from build123d import *

# Parameters (mm, degrees)
SKETCH1_W           = 30
SKETCH1_H           = 29
BOSS_EXTRUDE1_DEPTH = 10
SKETCH2_W           = 4
SKETCH2_H           = 10
CUT_EXTRUDE1_DEPTH  = 10
CHAMFER1_SIZE       = 4
SKETCH3_R           = 2
CUT_EXTRUDE2_DEPTH  = 15
CHAMFER2_SIZE       = 0.5
SKETCH4_R           = 10
CUT_EXTRUDE3_DEPTH  = 24.135470603
BOSS_EXTRUDE2_DEPTH = 19
CHAMFER3_SIZE       = 4
SKETCH6_W           = 28
SKETCH6_H           = 10
CUT_EXTRUDE4_DEPTH  = 15
FILLET1_R           = 5
SKETCH7_R           = 1.75
CUT_EXTRUDE5_DEPTH  = 69.85245211
FILLET2_R           = 2
SKETCH8_R           = 2
CUT_EXTRUDE6_DEPTH  = 61.478592634
SKETCH9_R           = 7.5
CUT_EXTRUDE7_DEPTH  = 5
BOSS_EXTRUDE3_DEPTH = 5


with BuildPart() as part:
    # Sketch1 → Boss-Extrude1 (new body)
    with BuildSketch(Plane.XY):
        Rectangle(SKETCH1_W, SKETCH1_H)
    extrude(amount=BOSS_EXTRUDE1_DEPTH)

    # Sketch2 → Cut-Extrude1 (cut)
    with BuildSketch(Plane.XZ.offset(14.5)):
        with Locations((-13, 5)):
            Rectangle(SKETCH2_W, SKETCH2_H)
        with Locations((13, 5)):
            Rectangle(SKETCH2_W, SKETCH2_H)
    extrude(amount=-CUT_EXTRUDE1_DEPTH, mode=Mode.SUBTRACT)

    # Chamfer1
    chamfer1_edges = [part.edges().sort_by_distance(p)[0] for p in [
        (11, -4.5, 5),
        (-11, -4.5, 5),
    ]]
    chamfer(chamfer1_edges, length=CHAMFER1_SIZE - 0.0001)  # a hair under: the kernel refuses the full size

    # Sketch3 → Cut-Extrude2 (cut)
    with BuildSketch(Plane.XZ.offset(14.5)):
        with Locations(Location((-7.5, 5, 0), (0, 0, 270))):
            Circle(SKETCH3_R)
        with Locations(Location((0, 5, 0), (0, 0, 270))):
            Circle(SKETCH3_R)
        with Locations(Location((7.5, 5, 0), (0, 0, 270))):
            Circle(SKETCH3_R)
    extrude(amount=-CUT_EXTRUDE2_DEPTH, mode=Mode.SUBTRACT)

    # Chamfer2
    chamfer2_edges = [part.edges().sort_by_distance(p)[0] for p in [
        (-7.5, -14.5, 7),
        (0, -14.5, 7),
        (7.5, -14.5, 7),
    ]]
    chamfer(chamfer2_edges, length=CHAMFER2_SIZE)

    # Sketch4 → Cut-Extrude3 (cut, through all)
    with BuildSketch(Plane(origin=(0, 0, 0), x_dir=(-1, 0, 0), z_dir=(0, 0, -1))):
        with Locations((0, -2.5)):
            Circle(SKETCH4_R)
    extrude(amount=-CUT_EXTRUDE3_DEPTH, mode=Mode.SUBTRACT)

    # Sketch5 → Boss-Extrude2 (add, symmetric)
    with BuildSketch(Plane(origin=(0, 0, 0), x_dir=(0, 0, -1), z_dir=(1, 0, 0))):
        Polygon((-10, 13.5), (-27.320508076, 23.5), (-27.320508076, 50.5), (-17.320508076, 50.5), (-17.320508076, 24.5), (0, 14.5), align=None)
    extrude(amount=BOSS_EXTRUDE2_DEPTH, both=True)

    # Chamfer3
    chamfer3_edges = [part.edges().sort_by_distance(p)[0] for p in [
        (-19, 14, 5),
        (19, 14, 5),
    ]]
    chamfer(chamfer3_edges, length=CHAMFER3_SIZE - 0.0001)  # a hair under: the kernel refuses the full size

    # Sketch6 → Cut-Extrude4 (cut)
    with BuildSketch(Plane(origin=(0, 50.5, 0), x_dir=(1, 0, 0), z_dir=(0, 1, 0))):
        with Locations((0, -22.320508076)):
            Rectangle(SKETCH6_W, SKETCH6_H)
    extrude(amount=-CUT_EXTRUDE4_DEPTH, mode=Mode.SUBTRACT)

    # Fillet1
    fillet1_edges = [part.edges().sort_by_distance(p)[0] for p in [
        (16.5, 50.5, 17.320508076),
        (16.5, 50.5, 27.320508076),
        (-16.5, 50.5, 17.320508076),
        (-16.5, 50.5, 27.320508076),
    ]]
    fillet(fillet1_edges, radius=FILLET1_R - 0.0001)  # a hair under: the kernel refuses the full size

    # Sketch7 → Cut-Extrude5 (cut, through all)
    with BuildSketch(Plane(origin=(19, 0, 0), x_dir=(0, 0, -1), z_dir=(1, 0, 0))):
        with Locations((-22.320508076, 45.5)):
            Circle(SKETCH7_R)
    extrude(amount=-CUT_EXTRUDE5_DEPTH, mode=Mode.SUBTRACT)

    # Fillet2
    fillet2_edges = [part.edges().sort_by_distance(p)[0] for p in [
        (19, 34.50005, 27.320508076),
        (19, 49.035563195, 25.856071271),
        (19, 49.035563195, 18.78494488),
        (-19, 34.50005, 27.320508076),
        (-19, 49.035563195, 25.856071271),
        (-19, 49.035563195, 18.78494488),
        (-19, 35.00005, 17.320508076),
        (19, 35.00005, 17.320508076),
    ]]
    fillet(fillet2_edges, radius=FILLET2_R)

    # Sketch8 → Cut-Extrude6 (cut, through all)
    with BuildSketch(Plane.XY.offset(27.320508076)):
        with Locations((0, 30.5)):
            Circle(SKETCH8_R)
    extrude(amount=-CUT_EXTRUDE6_DEPTH, mode=Mode.SUBTRACT)

    # Sketch9 → Cut-Extrude7 (cut)
    with BuildSketch(Plane.XY.offset(27.320508076)):
        with Locations((0, 30.5)):
            Circle(SKETCH9_R)
    extrude(amount=-CUT_EXTRUDE7_DEPTH, mode=Mode.SUBTRACT)

    # Sketch10 → Boss-Extrude3 (add)
    with BuildSketch(Plane(origin=(15, 0, 0), x_dir=(0, 0, -1), z_dir=(1, 0, 0))):
        Polygon((-10, -4.5), (-25.320508076, 22.345299462), (-10, 13.5), align=None)
    boss_extrude3 = extrude(amount=-BOSS_EXTRUDE3_DEPTH)

    # Mirror1: Boss-Extrude3 across plane
    add(boss_extrude3.mirror(Plane(origin=(0, 0, 0), x_dir=(0, 0, 1), z_dir=(1, 0, 0))))


solid = part.part
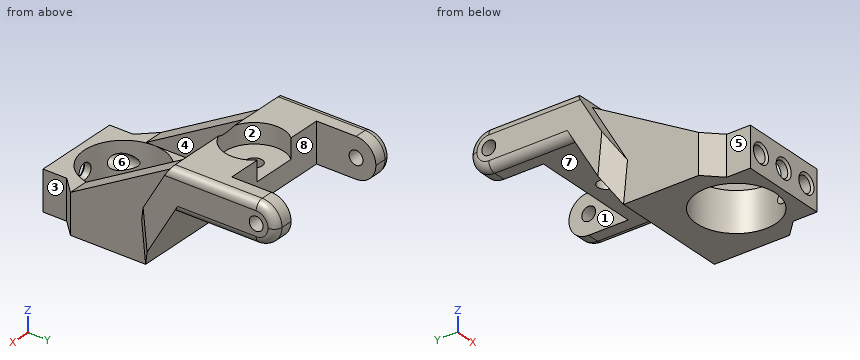
The listing builds one solid part. Answer for the finished solid, in the listing's coordinates (mm). Face numbers are marked on the shaded views. A direction names the side the tool comes from. Coordinates: 2 decimals unless noted, no trailing zeros. Loops run counter-clockwise (first coordinate to the right, second up) from the corner with the lowest first, then second, coordinate; pieces in that order, holes last. Notation, with made-up numbers: (25.25, 39.25) -> (72.25, 39.25) arc R25 ccw to (72.25, 77.25) -> close; hole circle Ø9 at (74, 65.5). An arc over 180 degrees is marked (long way). Answer in a Markdown table with one row per item. Add a question column.
1. Determine the mould class of the marked faces 6, 7 and 8 for opening direction Z: +Z half, -Z half, draft (parallel to the pull), parting line (faces both ways), or undercut.
2. The part is cut by section D-D, the plane y = 41.5. Write down the section's boundary in (x, z).
3. The part is cut by section A-A, the plane y = 30.5. Write down the section's boundary in (x, z).
4. The part is cut by section B-B, the plane x = 3.5. Write down the section's boundary in (y, z), then the cut area to 3 significant figures.
5. Consider line 1 (X direction, y = -9.75, z = 5); line 2 (Z direction, x = 0, y = -13.3); line 3 (X direction, y = -7.5, z = 5). Determine where each line is inside the solid, lowest interval first. Write a range as [from, to].
6. Flat-ended cylindrical pins translate along their axes: P1, Ø8, axis at x = 12.5, z = 16, coming from the +Y side; P2, Ø10, axis at y = 4, z = 9, coming from the +X side; P3, Ø11, axis at x = 6.5, z = 23, coming from the +Y side. Find the tip coordinate at first contact, or state that the pin passes through.
7. The part is cut by section C-C, the plane z = 5. Count the separate pieces of the cut face and the enclosed holes in it, then the cut area to 3 significant figures.
8. For the marked faces 1, 2, 3, 4 and 5, determine the directions among +Z, -Z, +X, -X, +Y, -Y from which every point of the face is accessible in a straight line to the end or side of a thin tool.
Answer below:
| question | item | result |
|---|---|---|
| 1 | face 6 | undercut |
| 1 | face 7 | -Z half |
| 1 | face 8 | draft |
| 2 | outline | (-19, 19.32) arc R2 ccw to (-17, 17.32) -> (-14, 17.32) -> (-14, 27.32) -> (-17, 27.32) arc R2 ccw to (-19, 25.32) -> close; (14, 17.32) -> (17, 17.32) arc R2 ccw to (19, 19.32) -> (19, 25.32) arc R2 ccw to (17, 27.32) -> (14, 27.32) -> close |
| 3 | outline | (-19, 19.32) arc R2 ccw to (-17, 17.32) -> (-2, 17.32) -> (-2, 22.32) -> (-7.5, 22.32) -> (-7.5, 27.32) -> (-17, 27.32) arc R2 ccw to (-19, 25.32) -> close; (2, 17.32) -> (17, 17.32) arc R2 ccw to (19, 19.32) -> (19, 25.32) arc R2 ccw to (17, 27.32) -> (7.5, 27.32) -> (7.5, 22.32) -> (2, 22.32) -> close |
| 4 | outline | (-14.5, 0) -> (-11.87, 0) -> (-11.87, 10) -> (-14.5, 10) -> close; (6.87, 0) -> (14.5, 0) -> (24.5, 17.32) -> (35.5, 17.32) -> (35.5, 22.32) -> (23.87, 22.32) -> (23.87, 27.32) -> (23.5, 27.32) -> (13.5, 10) -> (6.87, 10) -> close |
| 4 | area | 272 mm2 |
| 5 | line 1 | [-11, -9.5], [9.5, 11] |
| 5 | line 2 | [0, 3], [7, 10] |
| 5 | line 3 | [-12, -9.5], [9.5, 12] |
| 6 | P1 | y = 49.76 |
| 6 | P2 | x = 15 |
| 6 | P3 | y = 35.5 |
| 7 | separate pieces | 3 |
| 7 | enclosed holes | 0 |
| 7 | area | 536 mm2 |
| 8 | face 1 | +Z, -Z, +Y |
| 8 | face 2 | +Z |
| 8 | face 3 | +Z, -Z, +X, -Y |
| 8 | face 4 | +Z, -Y |
| 8 | face 5 | +Z, -Z, -X, -Y |
